Input: part model. Units: mm. Frame: model coordinates. A direction names the side the tool comes from. Give positions to 0.01 mm unless a question says otherwise; leave off trailing zeros. Loops run counter-clockwise (first coordinate to the right, second up) from the corner with the lowest first, then second, coordinate; pieces in that order, holes last. Notation, with made-up numbers: (80, -8) - (118, -8) arc R23 cw to (118, 7) - close; hole circle Ø9 at (17.5, 38.5). An arc over 180 degrees is marked (long way). Answer as a JSON object with one key per item and string values.
from build123d import *

# Parameters (mm, degrees)
SKETCH_1_W          = 74
SKETCH_1_H          = 45
EXTRUDE_1_DEPTH     = 5
FILLET_1_R          = 10
FILLET_2_R          = 10
EXTRUDE_3_DEPTH     = 33
EXTRUDE_4_DEPTH     = 33
SKETCH_6_W          = 13
SKETCH_6_H          = 13
CUT_EXTRUDE_1_DEPTH = 60.282099079
CUT_EXTRUDE_3_DEPTH = 28
EXTRUDE_5_DEPTH     = 33
SKETCH_10_W         = 3
SKETCH_10_H         = 11.5
CUT_EXTRUDE_4_DEPTH = 28
SKETCH_11_R         = 1.6
CUT_EXTRUDE_5_DEPTH = 10


with BuildPart() as part:
    # 草图1 → 凸台-拉伸1 (new body)
    with BuildSketch(Plane.XY):
        Rectangle(SKETCH_1_W, SKETCH_1_H)
    extrude(amount=EXTRUDE_1_DEPTH)

    # 圆角1
    fillet_1_edges = [part.edges().sort_by_distance(p)[0] for p in [
        (-37, -22.5, 2.5),
    ]]
    fillet(fillet_1_edges, radius=FILLET_1_R)

    # 圆角2
    fillet_2_edges = [part.edges().sort_by_distance(p)[0] for p in [
        (37, -22.5, 2.5),
    ]]
    fillet(fillet_2_edges, radius=FILLET_2_R)

    # 草图4 → 凸台-拉伸3 (add)
    with BuildSketch(Plane.XY.offset(5)):
        Polygon((-35.261752955, -18.134131531), (-21.914141487, 4.984609691), (-10.309401077, -1.715390309), (-22.309401077, -22.5), (-20, -22.5), (-7.577350269, -0.983339502), (-22.646192295, 7.716660498), (-36.356272702, -16.029895342), align=None)
        Polygon((36.356272702, -16.029895342), (35.261752955, -18.134131531), (21.914141487, 4.984609691), (10.309401077, -1.715390309), (22.309401077, -22.5), (20, -22.5), (7.577350269, -0.983339502), (22.646192295, 7.716660498), align=None)
    extrude(amount=EXTRUDE_3_DEPTH)

    # 草图5 → 凸台-拉伸4 (add)
    with BuildSketch(Plane.XY.offset(5)):
        Polygon((-7.577350269, -0.983339502), (7.577350269, -0.983339502), (9.309401077, -3.983339502), (-9.309401077, -3.983339502), align=None)
    extrude(amount=EXTRUDE_4_DEPTH)

    # 草图6 → 切除-拉伸1 (cut, through all)
    with BuildSketch(Plane.XZ.offset(3.983339502)):
        with Locations((0.190598923, 29)):
            Rectangle(SKETCH_6_W, SKETCH_6_H)
        with Locations((0.190598923, 11.5)):
            Rectangle(SKETCH_6_W, SKETCH_6_H)
    extrude(amount=-CUT_EXTRUDE_1_DEPTH, mode=Mode.SUBTRACT)

    # 草图8 → 切除-拉伸3 (cut)
    with BuildSketch(Plane.XY.offset(38)):
        Polygon((-29.646192295, -4.407695155), (-24.146192295, 5.118584287), (-22.414141487, 4.118584287), (-27.914141487, -5.407695155), align=None)
        Polygon((27.914141487, -5.407695155), (29.646192295, -4.407695155), (24.146192295, 5.118584287), (22.414141487, 4.118584287), align=None)
    extrude(amount=-CUT_EXTRUDE_3_DEPTH, mode=Mode.SUBTRACT)

    # 草图9 → 凸台-拉伸5 (add)
    with BuildSketch(Plane.XY.offset(5)):
        Polygon((-34, 22.5), (-37, 22.5), (-37, -12.5), (-36.638694465, -15.163750927), (-36.356272702, -16.029895342), (-34, -11.948711306), align=None)
        Polygon((36.356272702, -16.029895342), (34, -11.948711306), (34, 22.5), (37, 22.5), (36.837751954, -14.294055877), align=None)
    extrude(amount=EXTRUDE_5_DEPTH)

    # 草图10 → 切除-拉伸4 (cut)
    with BuildSketch(Plane.XY.offset(38)):
        with Locations((-35.5, 4.75)):
            Rectangle(SKETCH_10_W, SKETCH_10_H)
        with Locations((35.5, 4.75)):
            Rectangle(SKETCH_10_W, SKETCH_10_H)
    extrude(amount=-CUT_EXTRUDE_4_DEPTH, mode=Mode.SUBTRACT)

    # 草图11 → 切除-拉伸5 (cut)
    with BuildSketch(Plane.XY.offset(5)):
        with Locations((-27, 18.5)):
            Circle(SKETCH_11_R)
        with Locations((0, 18.5)):
            Circle(SKETCH_11_R)
        with Locations((27, 18.5)):
            Circle(SKETCH_11_R)
    extrude(amount=-CUT_EXTRUDE_5_DEPTH, mode=Mode.SUBTRACT)


solid = part.part
Item 1: Access query for faces 1 (the face through (0, -3, 18)), 2 (the face through (-36, 10.5, 24)), 3 (the face through (-23.292, 4.626, 24.196)). Directions: +Z, -Z, +X, -X, +Y, -Y. A direction counts if a zero-diameter tool reaches every point of the face in a straight line with its end or side. Return the directions, or none.
Geometry check:
{"face 1": "+Y, -Y", "face 2": "+Z, +X, -X", "face 3": "+Z, -X, -Y"}
Item 2: Material intervals for line 1 (X direction, y = 13, z = 11.5); line 2 (Y direction, x = -27, z = 4); line 3 (X direction, y = -5, z = 11), sorted ascending. Write a range as [from, to].
Geometry check:
{"line 1": "x = [-37, -34], [34, 36.96]", "line 2": "y = [-22.5, 16.9], [20.1, 22.5]", "line 3": "x = [-37, -34], [-29.99, -28.62], [-12.21, -9.9], [9.9, 12.21], [28.62, 29.99], [34, 36.88]"}
Item 3: Contact query for flat-ended pins moving along their axis: P1, Ø7.5, axis at x = -19, y = -13.5, coming from the +Z side; P2, Ø2.5, axis at y = -2, z = 8.5, coming from the +X side; P3, Ø8, axis at x = -26, y = 1, coming from the +Z side; P4, Ø8, axis at x = 15, z = 17.5, coming from the -Y side. Output: stop coordinate, or through.
Geometry check:
{"P1": "stops at z = 38", "P2": "stops at x = 36.9", "P3": "stops at z = 10", "P4": "stops at y = -20.77"}
Item 4: Mould query, pull axis Y, two halves, no side actions, for faces 4 (the face through (-16.225, -11.962, 21.269)), 5 (the face through (23.292, 4.626, 24.196)), 6 (the face through (23, -9, 5)), 7 (the face through (-34, -3, 21)). Classes: released by +Y, released by -Y, zero draft, split by the parting line, or undercut.
Geometry check:
{"face 4": "undercut", "face 5": "released by -Y", "face 6": "undercut", "face 7": "zero draft"}
Item 5: Cut plane C-C (y = 18.5). Give the number of separate pieces and of enclosed holes in the cut face, then the cut area to 3 significant figures.
Geometry check:
{"separate pieces": "4", "enclosed holes": "0", "area": "519 mm2"}
Item 6: Cut plane B-B (x = 0). Return loops of the section in (y, z).
Geometry check:
{"outline": "(-22.5, 0) - (16.9, 0) - (16.9, 5) - (-22.5, 5) - close; (-3.98, 18) - (-0.98, 18) - (-0.98, 22.5) - (-3.98, 22.5) - close; (-3.98, 35.5) - (-0.98, 35.5) - (-0.98, 38) - (-3.98, 38) - close; (20.1, 0) - (22.5, 0) - (22.5, 5) - (20.1, 5) - close"}
Item 7: Cut plane D-D (y = 0). Return loops of the section in (x, z), then the cut area to 3 significant figures.
Geometry check:
{"outline": "(-37, 0) - (37, 0) - (37, 5) - (36.9, 5) - (36.9, 10) - (34, 10) - (34, 5) - (27.1, 5) - (27.1, 10) - (24.79, 10) - (24.79, 5) - (13.28, 5) - (13.28, 38) - (9.28, 38) - (9.28, 5) - (-9.28, 5) - (-9.28, 38) - (-13.28, 38) - (-13.28, 5) - (-24.79, 5) - (-24.79, 10) - (-27.1, 10) - (-27.1, 5) - (-34, 5) - (-34, 10) - (-37, 10) - close", "area": "687 mm2"}
